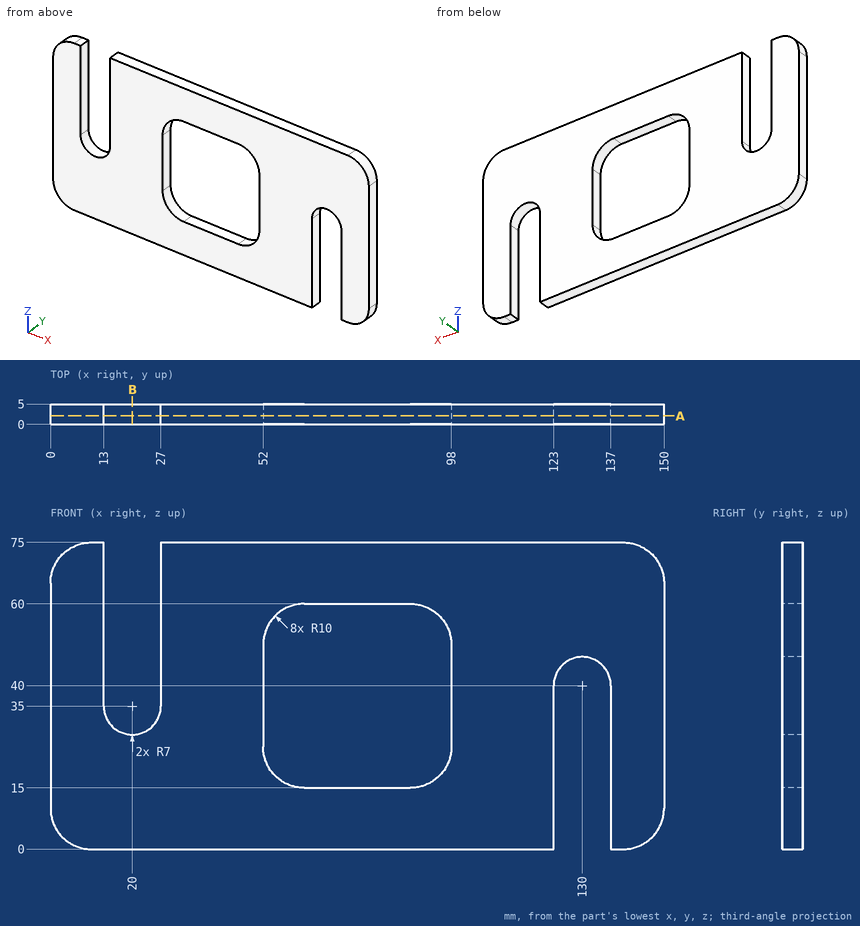
Could you check a few things on this drawing? It's one solid part, dimensions in mm from its lowest x, y, z. Give positions to 0.01 mm unless a question says otherwise; leave off trailing zeros. Write each loop counter-clockwise with the first axis right and the second up, starting at its lowest first coordinate (ties: lowest second). Pieces come first, ordered by that corner, then holes. Notation, with made-up numbers: (8.5, 6) - (12.5, 6) arc R19 ccw to (12.5, 29) - close; hole circle Ø10 at (37, 8). An arc over 180 degrees is marked (long way). Use CSV: the item, a comma, the result in double quotes. Start each with the question number.
Item 1: I want a section at A-A, the plane y = 2.1. Please give me the cut outline in (x, z), then the cut area to 3 significant figures.
Item 2: I want a section at B-B, the plane x = 20. Please give me the cut outline in (y, z), then the cut area to 3 significant figures.
Item 3: If I drill on line 1 along X through (y, z) = (3.6, 26); line 2 along X through (y, z) = (2.7, 13); line 3 along X through (y, z) = (0.8, 53), over which ranges is the centre line in solid material (lowest first)?
Item 4: I'm going to push a flat-ended pin straight in: pin 1 (6 mm diameter, centred on x = 127, z = 9, fed in from +Y). Where does the tip first touch, or does it pass through?
Findings:
1,outline,"(0, 10) arc R10 ccw to (10, 0) - (123, 0) - (123, 40) arc R7 cw to (137, 40) - (137, 0) - (140, 0) arc R10 ccw to (150, 10) - (150, 65) arc R10 ccw to (140, 75) - (27, 75) - (27, 35) arc R7 cw to (13, 35) - (13, 75) - (10, 75) arc R10 ccw to (0, 65) - close; hole (52, 25) arc R10 ccw to (62, 15) - (88, 15) arc R10 ccw to (98, 25) - (98, 50) arc R10 ccw to (88, 60) - (62, 60) arc R10 ccw to (52, 50) - close"
1,area,"7,910 mm2"
2,outline,"(0, 0) - (5, 0) - (5, 28) - (0, 28) - close"
2,area,"140 mm2"
3,line 1,"x = 0 to 52, 98 to 123, 137 to 150"
3,line 2,"x = 0 to 123, 137 to 150"
3,line 3,"x = 0 to 13, 27 to 52.46, 97.54 to 150"
4,pin 1,"passes through"
